Answer from the drawing. Dimensions are ordinates in mm from the lowest x, y and z of the part. A direction names the side the tool comes from. Round coordinates to 2 decimals unless told otherwise and drop trailing zeros. Loops run counter-clockwise (first coordinate to the right, second up) from the corner with the lowest first, then second, coordinate; pieces in that order, holes last. Notation, with made-up numbers: (21, 62) -> (55, 62) arc R36 cw to (55, 96) -> close; hole circle Ø4 at (-4, 84.5). An arc over 180 degrees is marked (long way). One line per question, with ' | ' between items.
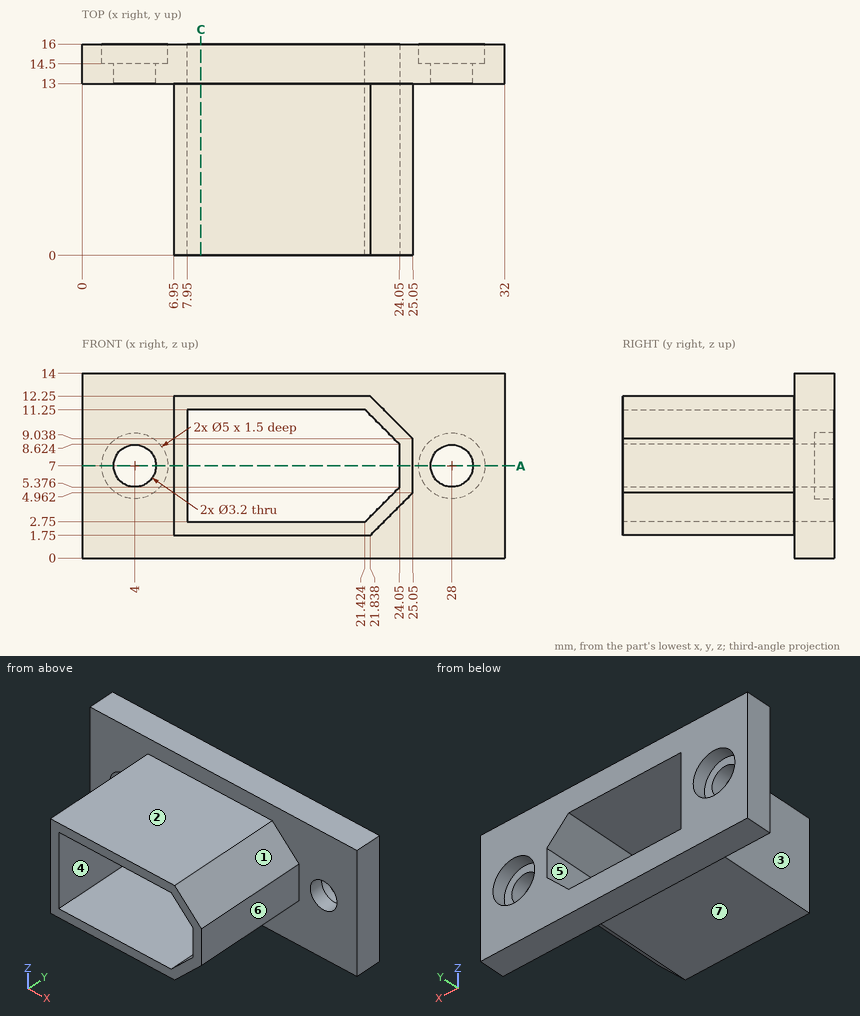
Q1. For a pull along X with two mould halves and no side action, classify the marked faces 5, 6 and 7 as pulls with the +X half, pulls with the -X half, needs draft (parallel to the pull), parting line crosses it, or undercut.
Numbers:
face 5: undercut | face 6: pulls with the +X half | face 7: needs draft
Q2. A cutting plane is placed at A-A on z = 7. Give the vertices of the cut face in (x, y).
Numbers:
outline: (0, 13) -> (2.4, 13) -> (2.4, 14.5) -> (1.5, 14.5) -> (1.5, 16) -> (0, 16) -> close; (5.6, 13) -> (6.95, 13) -> (6.95, 0) -> (7.95, 0) -> (7.95, 16) -> (6.5, 16) -> (6.5, 14.5) -> (5.6, 14.5) -> close; (24.05, 0) -> (25.05, 0) -> (25.05, 13) -> (26.4, 13) -> (26.4, 14.5) -> (25.5, 14.5) -> (25.5, 16) -> (24.05, 16) -> close; (29.6, 13) -> (32, 13) -> (32, 16) -> (30.5, 16) -> (30.5, 14.5) -> (29.6, 14.5) -> close
Q3. Find the intervals of material crossed by line 1 (X direction, y = 15.55, z = 7); line 2 (X direction, y = 13.8, z = 7); line 3 (Z direction, x = 12.5, y = 9.75), in increasing order. Write a range as from..to.
Numbers:
line 1: 0..1.5, 6.5..7.95, 24.05..25.5, 30.5..32 | line 2: 0..2.4, 5.6..7.95, 24.05..26.4, 29.6..32 | line 3: 1.75..2.75, 11.25..12.25
Q4. For the marked faces 1, 2, 3 and 4, determine the directions among +Z, -Z, +X, -X, +Y, -Y from which every point of the face is accessible in a straight line to the end or side of a thin tool.
Numbers:
face 1: +Z, +X, -Y | face 2: +Z, +X, -X, -Y | face 3: +Z, -Z, -X, -Y | face 4: +Y, -Y
Q5. Given pin 1 Ø2 at (y, z) = (3.5, 7) entering from +X; pin 2 Ø2.5 at (y, z) = (9, 7.5) entering from -X; pin 3 Ø3 at (x, z) = (5, 4) entering from -Y, each flat-ended and moving along its own axis, determine where each tip first touches the part or whether it passes through.
Numbers:
pin 1: x = 25.05 | pin 2: x = 6.95 | pin 3: y = 13
Q6. A cutting plane is placed at C-C on x = 9. Give the vertices of the cut face in (y, z).
Numbers:
outline: (0, 1.75) -> (13, 1.75) -> (13, 0) -> (16, 0) -> (16, 2.75) -> (0, 2.75) -> close; (0, 11.25) -> (16, 11.25) -> (16, 14) -> (13, 14) -> (13, 12.25) -> (0, 12.25) -> close
